Verification items for the finished model (mm, model axes). A direction names the side the tool comes from. Coordinates: 2 decimals unless noted, no trailing zeros. Order: outer loops, then holes, each group sorted by start corner. A loop starts at its lowest first (then second) coordinate and runs counter-clockwise, first axis right, second up.
Q1. Cross-section at C-C, the plane z = -1405. Record the boundary of the cut face in (x, y) (3 decimals).
Q2. Thickness scan on line 1 (Y direction, x = -6, z = -1488) (3 decimals). Record the ranges inside material, lowest first.
Q3. Draft check along X on faces 3 (the flat face through (0, -8.255, -1369)), 4 (the flat face through (-9, 0, -1524)), 5 (the flat face through (-9.525, 0, -1369)). Enter one of: pulls with the +X half, pulls with the -X half, needs draft (parallel to the pull), parting line crosses it, or undercut.
Q4. Cross-section at A-A, the plane y = -1.5. Record the boundary of the cut face in (x, z) (3 decimals), and give its area (3 significant figures).
Q5. Set-up check for faces 1 (the flat face through (8.255, 0, -1369)), 2 (the flat face through (0, -9, -1219.2)): record each of +Z, -Z, +X, -X, +Y, -Y from which the full face is reachable in a straight line by a thin tool's end or side.
from build123d import *

# Parameters (mm, degrees)
SKETCH1_W           = 19.05
SKETCH1_H           = 19.05
SKETCH1_W_2         = 16.51
SKETCH1_H_2         = 16.51
BOSS_EXTRUDE1_DEPTH = 1524
SKETCH2_W           = 2743.2
SKETCH2_H           = 19.05
CUT_EXTRUDE1_DEPTH  = 1525.148820859


with BuildPart() as part:
    # Sketch1 → Boss-Extrude1 (new, symmetric)
    with BuildSketch(Plane.XY):
        Rectangle(SKETCH1_W, SKETCH1_H)
        Rectangle(SKETCH1_W_2, SKETCH1_H_2, mode=Mode.SUBTRACT)
    extrude(amount=BOSS_EXTRUDE1_DEPTH, both=True)

    # Sketch2 → Cut-Extrude1 (cut, through all)
    with BuildSketch(Plane(origin=(9.525, 0, 0), x_dir=(0, 0, -1), z_dir=(1, 0, 0))):
        with Locations((-152.4, 0)):
            Rectangle(SKETCH2_W, SKETCH2_H)
    extrude(amount=-CUT_EXTRUDE1_DEPTH, mode=Mode.SUBTRACT)


solid = part.part
Check values:
1. outline: (-9.525, -9.525) - (9.525, -9.525) - (9.525, 9.525) - (-9.525, 9.525) - close; hole (-8.255, -8.255) - (8.255, -8.255) - (8.255, 8.255) - (-8.255, 8.255) - close
2. line 1: y = -9.525 to -8.255, 8.255 to 9.525
3. face 3: undercut
3. face 4: needs draft
3. face 5: pulls with the -X half
4. outline: (-9.525, -1524) - (-8.255, -1524) - (-8.255, -1219.2) - (-9.525, -1219.2) - close; (8.255, -1524) - (9.525, -1524) - (9.525, -1219.2) - (8.255, -1219.2) - close
4. area: 774 mm2
5. face 1: +Z, -Z
5. face 2: +Z, +X, -X, +Y, -Y
